Source: CAD feature listing. Evaluate the final solid. Frame: model axes, mm. A direction names the side the tool comes from. Round coordinates to 2 decimals unless told otherwise and drop trailing zeros. Loops run counter-clockwise (first coordinate to the right, second up) from the corner with the lowest first, then second, coordinate; pieces in that order, holes last. Notation, with made-up numbers: M 19,82.25 L 53,82.25 A21 cw 53,113.25 Z; hole C 73.5,25 d3. An arc over 180 degrees is marked long. Answer as a JSON object with one key per item and string values.
Autodesk Inventor part; units mm, degrees
ref_plane "YZ Plane" through (0, 0, 0) normal (1, 0, 0) x (0, 1, 0)
ref_plane "XZ Plane" through (0, 0, 0) normal (0, 1, 0) x (-1, 0, 0)
ref_plane "XY Plane" through (0, 0, 0) normal (0, 0, 1) x (1, 0, 0)
sketch "Sketch1" plane through (0, 0, 0) normal (0, 1, 0) x (-1, 0, 0)
  circle A0 centre (0, 0) radius 12.5
  circle A1 centre (0, 0) radius 38.5
  line L0 (-8.8388, 8.8388) -> (-27.2236, 27.2236)
  line L1 (8.8388, -8.8388) -> (27.2236, -27.2236)
  line L2 (8.8388, 8.8388) -> (27.2236, 27.2236)
  line L3 (-8.8388, -8.8388) -> (-27.2236, -27.2236)
  line L4 (0, 38.5) -> (0, 12.5)
  line L5 (0, -12.5) -> (0, -38.5)
  line L6 (38.5, 0) -> (12.5, 0)
  line L7 (-12.5, 0) -> (-38.5, 0)
  dimension "d0" = 25
  dimension "d2" = 26
sketch "Sketch22" plane through (0, 0, 0) normal (0, 1, 0) x (-1, 0, 0)
  circle A0 centre (0, 0) radius 12.5
  circle A1 centre (0, 0) radius 38.5
  line L0 (-8.8388, 8.8388) -> (-27.2236, 27.2236)
  line L1 (8.8388, -8.8388) -> (27.2236, -27.2236)
  line L2 (8.8388, 8.8388) -> (27.2236, 27.2236)
  line L3 (-8.8388, -8.8388) -> (-27.2236, -27.2236)
  line L4 (0, 38.5) -> (0, 12.5)
  line L5 (0, -12.5) -> (0, -38.5)
  line L6 (38.5, 0) -> (12.5, 0)
  line L7 (-12.5, 0) -> (-38.5, 0)
  circle A2 centre (0, 0) radius 12.5
  circle A3 centre (0, 0) radius 38.5
  line L8 (-8.8388, 8.8388) -> (-27.2236, 27.2236)
  line L9 (8.8388, -8.8388) -> (27.2236, -27.2236)
  line L10 (8.8388, 8.8388) -> (27.2236, 27.2236)
  line L11 (-8.8388, -8.8388) -> (-27.2236, -27.2236)
  line L12 (0, 38.5) -> (0, 12.5)
  line L13 (0, -12.5) -> (0, -38.5)
  line L14 (38.5, 0) -> (12.5, 0)
  line L15 (-12.5, 0) -> (-38.5, 0)
  dimension "d128" = 25
  dimension "d129" = 26
  dimension "d130" = 25
  dimension "d131" = 26
sketch "Sketch23" plane through (0, 0, 0) normal (0, 1, 0) x (-1, 0, 0)
  circle A0 centre (0, 0) radius 12.5
  circle A1 centre (0, 0) radius 38.5
  line L0 (-8.8388, 8.8388) -> (-27.2236, 27.2236)
  line L1 (8.8388, -8.8388) -> (27.2236, -27.2236)
  line L2 (8.8388, 8.8388) -> (27.2236, 27.2236)
  line L3 (-8.8388, -8.8388) -> (-27.2236, -27.2236)
  line L4 (0, 38.5) -> (0, 12.5)
  line L5 (0, -12.5) -> (0, -38.5)
  line L6 (38.5, 0) -> (12.5, 0)
  line L7 (-12.5, 0) -> (-38.5, 0)
  dimension "d132" = 25
  dimension "d133" = 26
sketch "Sketch24" plane through (0, 0, 0) normal (0, 1, 0) x (-1, 0, 0)
  circle A0 centre (0, 0) radius 12.5
  circle A1 centre (0, 0) radius 38.5
  line L0 (-8.8388, 8.8388) -> (-27.2236, 27.2236)
  line L1 (8.8388, -8.8388) -> (27.2236, -27.2236)
  line L2 (8.8388, 8.8388) -> (27.2236, 27.2236)
  line L3 (-8.8388, -8.8388) -> (-27.2236, -27.2236)
  line L4 (0, 38.5) -> (0, 12.5)
  line L5 (0, -12.5) -> (0, -38.5)
  line L6 (38.5, 0) -> (12.5, 0)
  line L7 (-12.5, 0) -> (-38.5, 0)
  dimension "d134" = 25
  dimension "d135" = 26
sketch "Sketch25" plane through (0, 0, 0) normal (0, 1, 0) x (-1, 0, 0)
  circle A0 centre (0, 0) radius 12.5
  circle A1 centre (0, 0) radius 38.5
  line L0 (-8.8388, 8.8388) -> (-27.2236, 27.2236)
  line L1 (8.8388, -8.8388) -> (27.2236, -27.2236)
  line L2 (8.8388, 8.8388) -> (27.2236, 27.2236)
  line L3 (-8.8388, -8.8388) -> (-27.2236, -27.2236)
  line L4 (0, 38.5) -> (0, 12.5)
  line L5 (0, -12.5) -> (0, -38.5)
  line L6 (38.5, 0) -> (12.5, 0)
  line L7 (-12.5, 0) -> (-38.5, 0)
  dimension "d136" = 25
  dimension "d137" = 26
sketch "Sketch26" plane through (0, 0, 0) normal (0, 1, 0) x (-1, 0, 0)
  circle A0 centre (0, 0) radius 12.5
  circle A1 centre (0, 0) radius 38.5
  line L0 (-8.8388, 8.8388) -> (-27.2236, 27.2236)
  line L1 (8.8388, -8.8388) -> (27.2236, -27.2236)
  line L2 (8.8388, 8.8388) -> (27.2236, 27.2236)
  line L3 (-8.8388, -8.8388) -> (-27.2236, -27.2236)
  line L4 (0, 38.5) -> (0, 12.5)
  line L5 (0, -12.5) -> (0, -38.5)
  line L6 (38.5, 0) -> (12.5, 0)
  line L7 (-12.5, 0) -> (-38.5, 0)
  dimension "d138" = 25
  dimension "d139" = 26
sketch "Sketch27" plane through (0, 0, 0) normal (0, 1, 0) x (-1, 0, 0)
  circle A0 centre (0, 0) radius 12.5
  circle A1 centre (0, 0) radius 38.5
  line L0 (-8.8388, 8.8388) -> (-27.2236, 27.2236)
  line L1 (8.8388, -8.8388) -> (27.2236, -27.2236)
  line L2 (8.8388, 8.8388) -> (27.2236, 27.2236)
  line L3 (-8.8388, -8.8388) -> (-27.2236, -27.2236)
  line L4 (0, 38.5) -> (0, 12.5)
  line L5 (0, -12.5) -> (0, -38.5)
  line L6 (38.5, 0) -> (12.5, 0)
  line L7 (-12.5, 0) -> (-38.5, 0)
  dimension "d140" = 25
  dimension "d141" = 26
sketch "Sketch28" plane through (0, 0, 0) normal (0, 1, 0) x (-1, 0, 0)
  circle A0 centre (0, 0) radius 12.5
  circle A1 centre (0, 0) radius 38.5
  line L0 (-8.8388, 8.8388) -> (-27.2236, 27.2236)
  line L1 (8.8388, -8.8388) -> (27.2236, -27.2236)
  line L2 (8.8388, 8.8388) -> (27.2236, 27.2236)
  line L3 (-8.8388, -8.8388) -> (-27.2236, -27.2236)
  line L4 (0, 38.5) -> (0, 12.5)
  line L5 (0, -12.5) -> (0, -38.5)
  line L6 (38.5, 0) -> (12.5, 0)
  line L7 (-12.5, 0) -> (-38.5, 0)
  dimension "d142" = 25
  dimension "d143" = 26
extrude "Extrusion20" add sketch "Sketch1" along normal blind 5 contours A0 L4 A1 L2
extrude "Extrusion21" add sketch "Sketch24" along normal blind 10 contours A0 L2 A1 L6
extrude "Extrusion22" add sketch "Sketch22" along normal blind 15 contours L6 A1 L1 A0
extrude "Extrusion23" add sketch "Sketch28" along normal blind 20 contours L1 A1 L5 A0
extrude "Extrusion24" add sketch "Sketch1" along normal blind 25 contours L5 A1 L3 A0
extrude "Extrusion25" add sketch "Sketch27" along normal blind 30 contours L3 A1 L7 A0
extrude "Extrusion26" add sketch "Sketch1" along normal blind 35 contours A0 L7 A1 L0
extrude "Extrusion27" add sketch "Sketch23" along normal blind 40 contours A0 L0 A1 L4
sketch "Sketch29" plane through (0, 0, 0) normal (0, -1, 0) x (1, 0, 0)
  point P0 (0, 0)
extrude "Extrusion28" cut sketch "Sketch26" along normal blind 5 contours L6 A1 L1 A0
extrude "Extrusion29" cut sketch "Sketch25" along normal blind 10 contours L1 A1 L5 A0
extrude "Extrusion30" cut sketch "Sketch1" along normal blind 15 contours L5 A1 L3 A0
extrude "Extrusion31" cut sketch "Sketch1" along normal blind 20 contours L3 A1 L7 A0
extrude "Extrusion32" cut sketch "Sketch1" along normal blind 25 contours A0 L7 A1 L0
extrude "Extrusion33" cut sketch "Sketch1" along normal blind 30 contours A0 L0 A1 L4
properties part number "DireccionEscalones"
Item 1: Section C-C on x = 29. Return the cut outline in (y, z).
Answer sheet:
{"outline": "M 20,-25.32 L 30,-25.32 L 30,0 L 35,0 L 35,25.32 L 25,25.32 L 25,0 L 20,0 Z"}
Item 2: Line query: probe 1 along Y at (x, z) = (3, -29.5); probe 2 along Z at (x, y) = (-9, 9.5); probe 3 along X at (y, z) = (26, 0). Output: solid intervals per line, ascending. Write a range as from..to.
Answer sheet:
{"probe 1": "y = 15..25", "probe 2": "z = -9..-8.67, 8.67..9", "probe 3": "x = 12.5..38.5"}
Item 3: Section A-A on x = -2.5. Return the cut outline in (y, z).
Answer sheet:
{"outline": "M 0,12.25 L 5,12.25 L 5,38.42 L 0,38.42 Z; M 10,-38.42 L 20,-38.42 L 20,-12.25 L 10,-12.25 Z"}
Item 4: Contact query for flat-ended pins moving along their axis: pin 1 Ø22 at (x, z) = (7, -18) entering from +Y; pin 2 Ø1.5 at (x, z) = (-8.5, 17.5) entering from +Y; pin 3 Ø5.5 at (y, z) = (12, -20.5) entering from +X. Output: stop coordinate, or through.
Answer sheet:
{"pin 1": "stops at y = 30", "pin 2": "stops at y = 5", "pin 3": "stops at x = 0"}
Item 5: Section D-D on y = 21. Return the cut outline in (x, z).
Answer sheet:
{"outline": "M 0,-38.5 A38.5 ccw 38.5,0 L 12.5,0 A12.5 cw 0,-12.5 Z"}
Item 6: Access query for faces 1 (the flat face through (11, 25, -23)), 2 (the flat face through (-23, 15, -10)), 3 (the flat face through (11, 30, 24)). Directions: +Z, -Z, +X, -X, +Y, -Y. A direction counts if a zero-diameter tool reaches every point of the face in a straight line with its end or side. Return the directions, or none.
Answer sheet:
{"face 1": "-Z, -X, +Y", "face 2": "+Z, -X, +Y", "face 3": "+Z, -X, -Y"}
Item 7: Section B-B on z = 1. Return the cut outline in (x, y).
Answer sheet:
{"outline": "M -38.49,0 L -12.46,0 L -12.46,10 L -38.49,10 Z; M 12.46,25 L 38.49,25 L 38.49,35 L 12.46,35 Z"}
